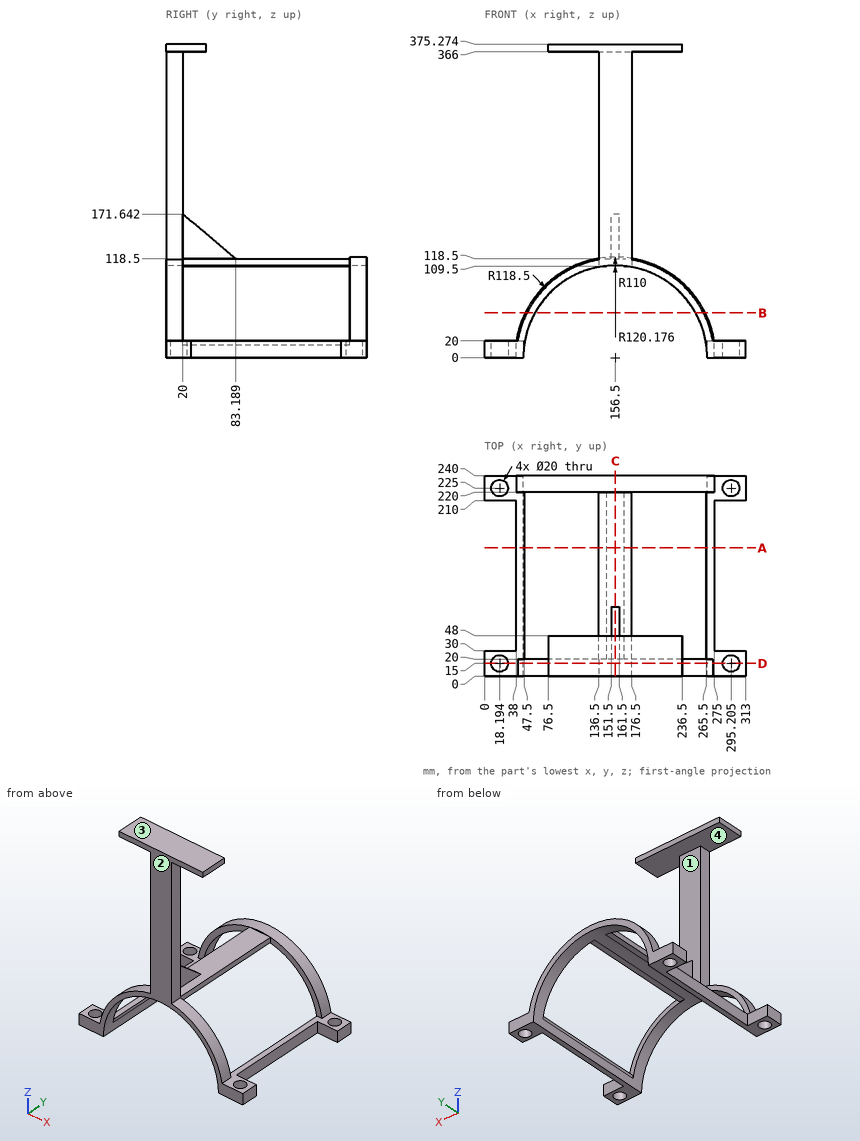
Here's the drawing with two shaded views (mm, measured from the low corner). I have some questions. Coordinates: 2 decimals unless noted, no trailing zeros. Loops run counter-clockwise (first coordinate to the right, second up) from the corner with the lowest first, then second, coordinate; pieces in that order, holes last.
Item 1: Suppose I cut it at C-C (x = 156.5). Please give me the cut outline in (y, z) (1 decimal), then the cut area to 3 significant figures.
Answers below:
outline: (0, 110) - (240, 110) - (240, 120.2) - (220, 120.2) - (220, 118.5) - (83.2, 118.5) - (20, 171.6) - (20, 366) - (48, 366) - (48, 375.3) - (0, 375.3) - close
area: 9,150 mm2
Item 2: Suppose I cut it at A-A (y = 153.5). Please give me the cut outline in (x, z), then the cut area to 3 significant figures.
Answers below:
outline: (38, 0) - (46.5, 0) arc R110 cw to (47.5, 14.8) - (47.5, 20) - (38, 20) - close; (136.5, 109.5) - (146.02, 109.5) arc R110 cw to (166.98, 109.5) - (176.5, 109.5) - (176.5, 118.5) - (136.5, 118.5) - close; (265.5, 14.8) arc R110 cw to (266.5, 0) - (275, 0) - (275, 20) - (265.5, 20) - close
area: 713 mm2
Item 3: If we mould it in two halves opening along Z, with no side actions, what happens to the marked faces 1, 2, 3 and 4? For each: released by +Z, released by -Z, zero draft, split by the parting line, or undercut.
Answers below:
face 1: undercut
face 2: zero draft
face 3: released by +Z
face 4: undercut
Item 4: Suppose I cut it at B-B (z = 53.5). Please give me the cut outline in (x, y) (1 decimal), then the cut area to 3 significant figures.
Answers below:
outline: (48.9, 220) - (60.4, 220) - (60.4, 240) - (48.9, 240) - close; (50.8, 0) - (60.4, 0) - (60.4, 20) - (50.8, 20) - close; (252.6, 0) - (262.2, 0) - (262.2, 20) - (252.6, 20) - close; (252.6, 220) - (264.1, 220) - (264.1, 240) - (252.6, 240) - close
area: 845 mm2
Item 5: Please list where these lines run through material, in increasing order: L1, parallel to Y at x = 72, z = 72; L2, parallel to Z at x = 273, y = 148; L3, parallel to Z at x = 223, y = 17 (1 decimal).
Answers below:
L1: y = 0 to 20, 220 to 240
L2: z = 0 to 20
L3: z = 87.6 to 98.1, 366 to 375.3
Item 6: I'm going to push flat-ended pins straight in: pin 1 (12 mm diameter, centred on x = 295.2, y = 225, fed in from -Z); pin 2 (4.5 mm diameter, centred on x = 118, z = 370.5, fed in from +Y); pin 3 (3 mm diameter, centred on y = 47, z = 121, fed in from +X); pin 4 (22 mm diameter, centred on y = 95.5, z = 8.5, fed in from +X). Where does each tip first touch, or does it pass through?
Answers below:
pin 1: passes through
pin 2: stops at y = 48
pin 3: stops at x = 161.5
pin 4: stops at x = 275
Item 7: Suppose I cut it at D-D (y = 15). Please give me the cut outline in (x, z) (1 decimal).
Answers below:
outline: (0, 0) - (8.2, 0) - (8.2, 20) - (0, 20) - close; (28.2, 0) - (46.5, 0) arc R110 cw to (266.5, 0) - (285.2, 0) - (285.2, 20) - (273.3, 20) arc R118.5 ccw to (176.5, 116.8) - (176.5, 366) - (236.5, 366) - (236.5, 375.3) - (76.5, 375.3) - (76.5, 366) - (136.5, 366) - (136.5, 116.8) arc R118.5 ccw to (39.7, 20) - (28.2, 20) - close; (305.2, 0) - (313, 0) - (313, 20) - (305.2, 20) - close
